Could you check a few things on this drawing? It's one solid part, dimensions in mm from its lowest x, y, z. A direction names the side the tool comes from. Give positions to 0.01 mm unless a question says otherwise; leave off trailing zeros. Order: outer loops, then holes, each group sorted by start corner. A loop starts at its lowest first (then second) coordinate and runs counter-clockwise, first axis right, second up. Notation, with made-up numbers: (68.5, 81) - (78.5, 81) arc R11 ccw to (78.5, 93) - close; hole circle Ø5 at (27.5, 46.5). An arc over 180 degrees is marked (long way). One line per question, with ' | ' between items. Start each with the question number.
1. Imagine slicing it at C-C (y = 7.75). Please give me the cut outline in (x, z).
2. For P1, Ø3, axis at x = 3.5, y = 7.5, coming from the +Z side; P2, Ø2, axis at x = 2, z = 19, coming from the -Y side (1 decimal); P3, Ø1, axis at x = 2, z = 10, coming from the +Y side (1 decimal), each with a flat end and sliding along its axis, tell me the tip position at first contact or that it passes through.
3. Imagine slicing it at B-B (z = 28). Please give me the cut outline in (x, y) (1 decimal).
4. I need wall thicknesses on probe 1 along Y at (x, z) = (7.75, 21) (1 decimal); probe 2 along Z at (x, y) = (2.5, 12.25) (1 decimal); probe 3 along Z at (x, y) = (3.75, 6) (1 decimal). Which ranges of each line are inside material? Lowest first, please. Write a range as from..to.
5. Which directions (+Z, -Z, +X, -X, +Y, -Y) give clear straight access to the entire face, cutting with the end or side of a thin tool? Please do the marked faces 1 and 2.
6. Imagine slicing it at A-A (x = 4.5). Please give me the cut outline in (y, z) (1 decimal).
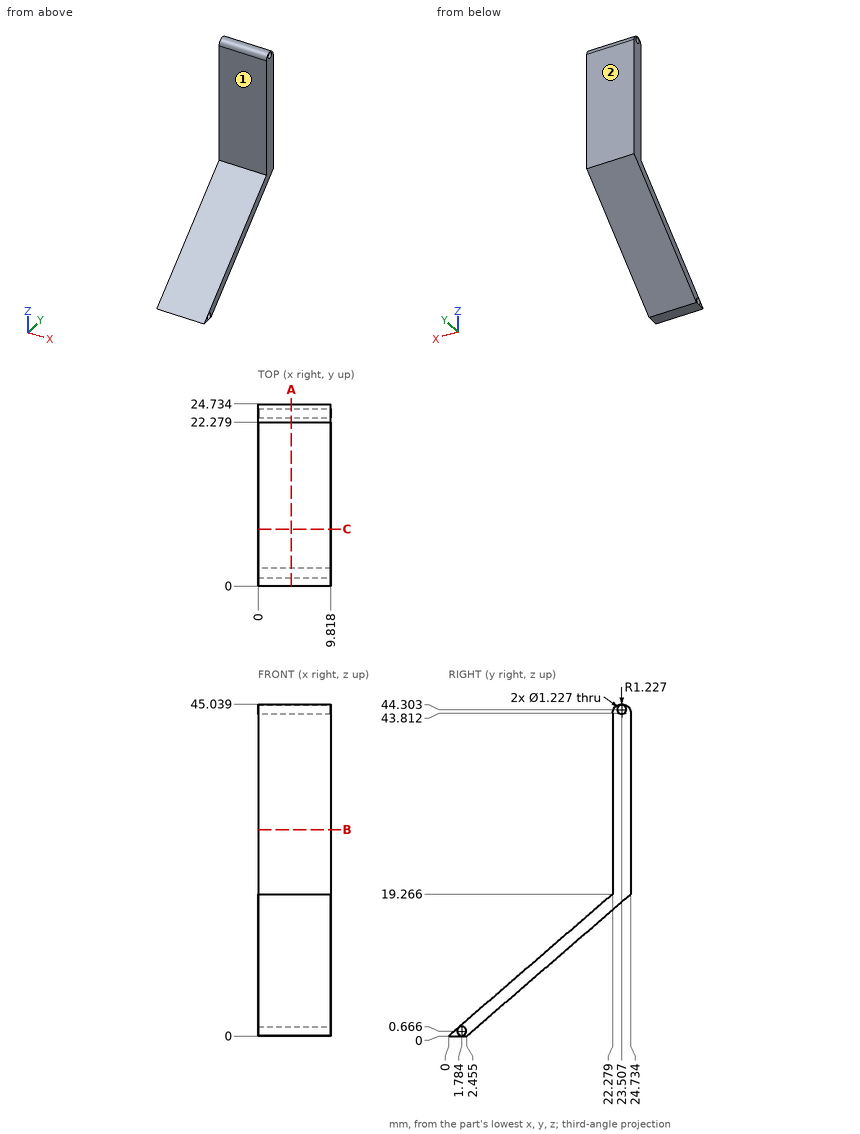
Results found:
1) outline: (0, 4.58) - (9.82, 4.58) - (9.82, 6.7) - (0, 6.7) - close
2) P1: stops at z = 7.78 | P2: stops at y = 20.8 | P3: stops at y = 14.6
3) outline: (0, 22.3) - (9.8, 22.3) - (9.8, 24.7) - (0, 24.7) - close
4) probe 1: y = 22.3..24.7 | probe 2: z = 8.5..10.6 | probe 3: z = 3.1..5.2
5) face 1: +Z, +X, -X, -Y | face 2: +Z, -Z, +X, -X, +Y
6) outline: (0, 0) - (2.5, 0) - (24.7, 19.3) - (24.7, 43.8) arc R1.2 ccw to (22.3, 43.8) - (22.3, 19.3) - close; hole circle Ø1.2 at (1.8, 0.7); hole circle Ø1.2 at (23.5, 44.3)
